The model under review builds one solid part; all positions refer to its coordinate system, in mm. Face numbers are marked on the shaded views. Give positions to 0.01 mm unless a question says otherwise; leave off trailing zeros. Order: outer loops, then holes, each group sorted by start corner. A loop starts at its lowest first (then second) coordinate and runs counter-clockwise, first axis right, second up.
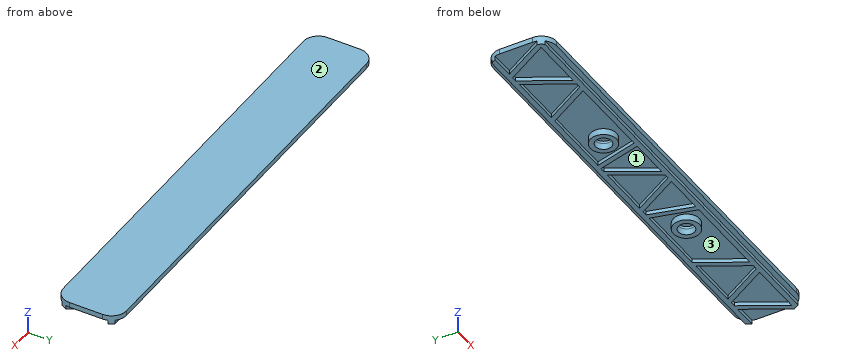
```python
from build123d import *

# Parameters (mm, degrees)
SKETCH1_W           = 173
SKETCH1_H           = 25
SKETCH1_R           = 3.2
BOSS_EXTRUDE1_DEPTH = 1
SKETCH2_W           = 173
SKETCH2_H           = 25
BOSS_EXTRUDE2_DEPTH = 1
SKETCH6_R           = 5.2
SKETCH6_R_2         = 3.2
BOSS_EXTRUDE5_DEPTH = 2.5
BOSS_EXTRUDE4_DEPTH = 1.5
FILLET1_R           = 6


with BuildPart() as part:
    # Sketch1 → Boss-Extrude1 (new body)
    with BuildSketch(Plane.XY):
        with Locations((27.85, 0)):
            Rectangle(SKETCH1_W, SKETCH1_H)
        Circle(SKETCH1_R, mode=Mode.SUBTRACT)
        with Locations((55.7, 0)):
            Circle(SKETCH1_R, mode=Mode.SUBTRACT)
    extrude(amount=-BOSS_EXTRUDE1_DEPTH)

    # Sketch2 → Boss-Extrude2 (add)
    with BuildSketch(Plane.XY):
        with Locations((27.85, 0)):
            Rectangle(SKETCH2_W, SKETCH2_H)
    extrude(amount=BOSS_EXTRUDE2_DEPTH)

    # Sketch6 → Boss-Extrude5 (add)
    with BuildSketch(Plane(origin=(0, 0, -1), x_dir=(-1, 0, 0), z_dir=(0, 0, -1))):
        with Locations(Location((-55.7, 0, 0), (0, 0, 180))):
            Circle(SKETCH6_R)
        with Locations(Location((-55.7, 0, 0), (0, 0, 180))):
            Circle(SKETCH6_R_2, mode=Mode.SUBTRACT)
        with Locations(Location((0, 0, 0), (0, 0, 180))):
            Circle(SKETCH6_R)
        with Locations(Location((0, 0, 0), (0, 0, 180))):
            Circle(SKETCH6_R_2, mode=Mode.SUBTRACT)
    extrude(amount=BOSS_EXTRUDE5_DEPTH)

    # Sketch5 → Boss-Extrude4 (add)
    with BuildSketch(Plane(origin=(0, 0, -1), x_dir=(-1, 0, 0), z_dir=(0, 0, -1))):
        Polygon((-27.85, -10.5), (-27.85, -8.5), (-28.85, -8.5), (-38.664954576, 8.5), (-27.85, 8.5), (-27.85, 10.5), (-114.35, 10.5), (-114.35, 8.5), (-104.535045424, 8.5), (-114.35, -8.5), (-114.35, -10.5), align=None)
        Polygon((-112.040598923, -8.5), (-90.410689771, -8.5), (-100.225644347, 8.5), (-102.225644347, 8.5), align=None, mode=Mode.SUBTRACT)
        Polygon((-97.91624327, 8.5), (-88.101288694, -8.5), (-86.101288694, -8.5), (-76.286334118, 8.5), align=None, mode=Mode.SUBTRACT)
        Polygon((-83.791887617, -8.5), (-73.976933041, 8.5), (-45.044908014, 8.5), (-49.600044285, -8.5), align=None, mode=Mode.SUBTRACT)
        Polygon((-40.974355653, 8.5), (-31.159401077, -8.5), (-47.529491924, -8.5), (-42.974355653, 8.5), align=None, mode=Mode.SUBTRACT)
    boss_extrude4 = extrude(amount=BOSS_EXTRUDE4_DEPTH)

    # Mirror1: Boss-Extrude4 across plane
    add(boss_extrude4.mirror(Plane(origin=(27.85, 0, 0), x_dir=(0, 0, 1), z_dir=(1, 0, 0))))

    # Fillet1
    fillet1_edges = [part.edges().sort_by_distance(p)[0] for p in [
        (114.35, 12.5, 0),
        (114.35, -12.5, 0),
        (-58.65, -12.5, 0),
        (-58.65, 12.5, 0),
    ]]
    fillet(fillet1_edges, radius=FILLET1_R)


solid = part.part
```
Item 1: Take a section at A-A (x = 0). Give the boundary of the cut face in (y, z), and give its area (3 significant figures).
Values found:
outline: (-12.5, -1) - (-10.5, -1) - (-10.5, -2.5) - (-8.5, -2.5) - (-8.5, -1) - (-5.2, -1) - (-5.2, -3.5) - (-3.2, -3.5) - (-3.2, 0) - (3.2, 0) - (3.2, -3.5) - (5.2, -3.5) - (5.2, -1) - (8.5, -1) - (8.5, -2.5) - (10.5, -2.5) - (10.5, -1) - (12.5, -1) - (12.5, 1) - (-12.5, 1) - close
area: 59.6 mm2
Item 2: Draft analysis for pull direction Y (two halves, no side actions). For the marked faces 1, 2 and 3, state which applies: released by +Y, released by -Y, zero draft, split by the parting line, or undercut.
Values found:
face 1: undercut
face 2: zero draft
face 3: undercut
Item 3: Clearance check with flat-ended pins moving along their axes: pin 1 Ø1.6 at (x, z) = (-46, -2) entering from -Y; pin 2 Ø13 at (x, y) = (41, 4) entering from -Z; pin 3 Ø8.5 at (x, y) = (55.7, 0) entering from -Z; pin 4 Ø0.8 at (x, z) = (29, -2) entering from +Y. State where each tip first meets the part, or that it passes through.
Values found:
pin 1: stops at y = -10.5
pin 2: stops at z = -2.5
pin 3: stops at z = -3.5
pin 4: stops at y = 10.5
Item 4: For line 1 (Y direction, x = 0, z = -1.65); line 2 (Y direction, x = 0, z = -2.6); line 3 (Z direction, x = 52, y = -9), list the stretches that pass through material, from the lowest coordinate up.
Values found:
line 1: y = -10.5 to -8.5, -5.2 to -3.2, 3.2 to 5.2, 8.5 to 10.5
line 2: y = -5.2 to -3.2, 3.2 to 5.2
line 3: z = -2.5 to 1
Item 5: Take a section at B-B (x = 68). Give the boundary of the cut face in (y, z), and give its area (3 significant figures).
Values found:
outline: (-12.5, -1) - (-10.5, -1) - (-10.5, -2.5) - (-8.5, -2.5) - (-8.5, -1) - (8.5, -1) - (8.5, -2.5) - (10.5, -2.5) - (10.5, -1) - (12.5, -1) - (12.5, 1) - (-12.5, 1) - close
area: 56.0 mm2
